Source: CAD feature listing. Evaluate the final solid. Frame: model axes, mm. A direction names the side the tool comes from. Round coordinates to 2 decimals unless told otherwise and drop trailing zeros. Order: outer loops, then holes, each group sorted by start corner. A loop starts at its lowest first (then second) coordinate and runs counter-clockwise, first axis right, second up.
Autodesk Inventor part; units mm, degrees
ref_plane "YZ Plane" through (0, 0, 0) normal (1, 0, 0) x (0, 1, 0)
ref_plane "XZ Plane" through (0, 0, 0) normal (0, 1, 0) x (-1, 0, 0)
ref_plane "XY Plane" through (0, 0, 0) normal (0, 0, 1) x (1, 0, 0)
sketch "Sketch1" plane through (0, 0, 0) normal (0, 0, 1) x (1, 0, 0)
  line L0 (-12, 21) -> (12, 21)
  line L1 (12, 21) -> (12, -21)
  line L2 (12, -21) -> (-12, -21)
  line L3 (-12, -21) -> (-12, 21)
  point P0 (0, 0)
  point P1 (12, 0)
  point P2 (0, 21)
  dimension "d0" = 24
  dimension "d1" = 42
extrude "Extrusion1" add sketch "Sketch1" along normal blind 34
sketch "Sketch2" plane through (0, 0, 34) normal (0, 0, 1) x (1, 0, 0)
  circle A0 centre (0, 0) radius 6.25
  dimension "d4" = 12.5
extrude "Extrusion2" add sketch "Sketch2" along normal blind 12
properties part number "s823switch"
1. Section D-D on y = 13.5. Return loops of the section in (x, z).
2. Line query: line 1 along Z through (x, y) = (-1, -8); line 2 along Y through (x, z) = (-5.75, 37); line 3 along X through (y, z) = (-1, 38.5). Output: solid intervals per line, ascending.
3. Section C-C on x = -7.5. Return loops of the section in (y, z), plus the area to 3 significant figures.
4. Section A-A on x = 0. Return loops of the section in (y, z), plus the area to 3 significant figures.
5. Section B-B on y = 0. Return loops of the section in (x, z), plus the area to 3 significant figures.
6. Access query for faces 1 (the face through (-12, 0, 17)), 2 (the face through (5.96, -1.88, 39.92)). Directions: +Z, -Z, +X, -X, +Y, -Y. A direction counts if a zero-diameter tool reaches every point of the face in a straight line with its end or side. Return the directions, or none.
7. First-contact query: pin 1 (10 mm diameter, centred on x = -2.5, z = 39.5, fed in from -Y); pin 2 (1 mm diameter, centred on x = 2.5, z = 36, fed in from +Y). Flat tips, straight axial feed; report the tip coordinate or a pass-through.
Result:
1. outline: (-12, 0) - (12, 0) - (12, 34) - (-12, 34) - close
2. line 1: z = 0 to 34
2. line 2: y = -2.45 to 2.45
2. line 3: x = -6.17 to 6.17
3. outline: (-21, 0) - (21, 0) - (21, 34) - (-21, 34) - close
3. area: 1,430 mm2
4. outline: (-21, 0) - (21, 0) - (21, 34) - (6.25, 34) - (6.25, 46) - (-6.25, 46) - (-6.25, 34) - (-21, 34) - close
4. area: 1,580 mm2
5. outline: (-12, 0) - (12, 0) - (12, 34) - (6.25, 34) - (6.25, 46) - (-6.25, 46) - (-6.25, 34) - (-12, 34) - close
5. area: 966 mm2
6. face 1: +Z, -Z, -X, +Y, -Y
6. face 2: +Z
7. pin 1: stops at y = -6.25
7. pin 2: stops at y = 5.92
